Build history of the part. All positions in model axes, mm. Round coordinates to 2 decimals unless told otherwise and drop trailing zeros. Loops run counter-clockwise (first coordinate to the right, second up) from the corner with the lowest first, then second, coordinate; pieces in that order, holes last. Notation, with made-up numbers: M 6,-12.5 L 44,-12.5 A23 cw 44,23.5 Z; hole C -14.75,-4 d7. An arc over 180 degrees is marked long. One line per item, written item: value.
```python
from build123d import *

# Parameters (mm, degrees)
SKETCH4_R           = 1.0999978
BOSS_EXTRUDE4_DEPTH = 3.175
SKETCH1_R           = 1.1999976
CUT_EXTRUDE7_DEPTH  = 62.35209393
CUT_EXTRUDE9_DEPTH  = 62.35209393
CIRPATTERN1_COUNT   = 3
SKETCH9_W           = 40.35933
SKETCH9_H           = 5.08
BOSS_EXTRUDE5_DEPTH = 3.175
SKETCH10_R          = 1.2
CUT_EXTRUDE10_DEPTH = 64.132493246
CIRPATTERN2_COUNT   = 3
FILLET3_R           = 20.32
FILLET4_R           = 2.54
SKETCH13_W          = 6.35
SKETCH13_H          = 6.35
CUT_EXTRUDE12_DEPTH = 63.881962359


with BuildPart() as part:
    # Sketch4 → Boss-Extrude4 (new body)
    with BuildSketch(Plane(origin=(0, 0, 0), x_dir=(1, 0, 0), z_dir=(0, 1, 0))):
        with BuildLine():
            Line((-19.99996, 34.84845233), (-40.179625, -0.10375273))
            ThreePointArc((-40.179625, -0.10375273), (-38.616778752, -22.295407608), (-20.179665, -34.744699599))
            Line((-20.179665, -34.744699599), (0, -34.744699599))
            Line((0, -34.744699599), (20.179665, -34.744699599))
            ThreePointArc((20.179665, -34.744699599), (38.616778752, -22.295407608), (40.179625, -0.10375273))
            Line((40.179625, -0.10375273), (30.0897925, 17.3723498))
            Line((30.0897925, 17.3723498), (19.99996, 34.84845233))
            ThreePointArc((19.99996, 34.84845233), (0, 44.590815215), (-19.99996, 34.84845233))
        make_face()
        with Locations(Location((-5.000000033, 0, 0), (0, 0, 270))):
            Circle(SKETCH4_R, mode=Mode.SUBTRACT)
        with Locations(Location((5.000000033, 0, 0), (0, 0, 270))):
            Circle(SKETCH4_R, mode=Mode.SUBTRACT)
    extrude(amount=BOSS_EXTRUDE4_DEPTH)

    # Sketch1 → Cut-Extrude7 (cut, through all)
    with BuildSketch(Plane(origin=(0, 3.175, 0), x_dir=(1, 0, 0), z_dir=(0, 1, 0))):
        with Locations(Location((10.835999918, -25.497765942, 0), (0, 0, 270))):
            Circle(SKETCH1_R)
        with Locations(Location((10.835999918, -7.497801942, 0), (0, 0, 270))):
            Circle(SKETCH1_R)
        with Locations(Location((-11.911286913, -5.635350233, 0), (0, 0, 270))):
            Circle(SKETCH1_R)
        with Locations(Location((-27.499713005, 3.364631767, 0), (0, 0, 270))):
            Circle(SKETCH1_R)
        with Locations(Location((1.075286995, 13.133152175, 0), (0, 0, 270))):
            Circle(SKETCH1_R)
        with Locations(Location((16.663713087, 22.133134175, 0), (0, 0, 270))):
            Circle(SKETCH1_R)
    extrude(amount=-CUT_EXTRUDE7_DEPTH, mode=Mode.SUBTRACT)

    # Sketch6 → Cut-Extrude9 (cut, through all)
    with BuildSketch(Plane(origin=(0, 3.175, 0), x_dir=(1, 0, 0), z_dir=(0, 1, 0))):
        with BuildLine():
            Line((-20.179665, -31.862440942), (20.179665, -31.862440942))
            ThreePointArc((20.179665, -31.862440942), (20.554442, -31.487663942), (20.179665, -31.112886942))
            Line((20.179665, -31.112886942), (-20.179665, -31.112886942))
            ThreePointArc((-20.179665, -31.112886942), (-20.554442, -31.487663942), (-20.179665, -31.862440942))
        make_face()
    cut_extrude9 = extrude(amount=-CUT_EXTRUDE9_DEPTH, mode=Mode.SUBTRACT)

    # CirPattern1: Cut-Extrude9 ×3 about axis
    cirpattern1_axis = Axis((0, 0, -0.195474675), (0, 1, 0))
    for i in range(1, CIRPATTERN1_COUNT):
        add(cut_extrude9.rotate(cirpattern1_axis, i * 360 / CIRPATTERN1_COUNT), mode=Mode.SUBTRACT)

    # Sketch9 → Boss-Extrude5 (add)
    with BuildSketch(Plane(origin=(0, 3.175, 0), x_dir=(1, 0, 0), z_dir=(0, 1, 0))):
        Polygon((-19.99996, 34.84845233), (-24.399369051, 37.38845233), (-44.579034051, 2.43624727), (-40.179625, -0.10375273), align=None)
        with Locations((0, -37.284699599)):
            Rectangle(SKETCH9_W, SKETCH9_H)
        Polygon((19.99996, 34.84845233), (24.399369051, 37.38845233), (44.579034051, 2.43624727), (40.179625, -0.10375273), align=None)
    extrude(amount=-BOSS_EXTRUDE5_DEPTH)

    # Sketch10 → Cut-Extrude10 (cut, through all)
    with BuildSketch(Plane(origin=(0, 3.175, 0), x_dir=(1, 0, 0), z_dir=(0, 1, 0))):
        with Locations(Location((-32.140098419, 18.556094474, 0), (0, 0, 270))):
            Circle(SKETCH10_R)
    cut_extrude10 = extrude(amount=-CUT_EXTRUDE10_DEPTH, mode=Mode.SUBTRACT)

    # CirPattern2: Cut-Extrude10 ×3 about axis
    cirpattern2_axis = Axis((0.026468548, 0, 0.018558184), (0, 1, 0))
    for i in range(1, CIRPATTERN2_COUNT):
        add(cut_extrude10.rotate(cirpattern2_axis, i * 360 / CIRPATTERN2_COUNT), mode=Mode.SUBTRACT)

    # Fillet3
    # the kernel refuses this fillet: 20.32 mm, written as the material it adds along each edge
    with BuildSketch(Plane(origin=(-19.99996, 0, -34.84845233), x_dir=(0.7399559261961443, 0, -0.6726553555032522), z_dir=(0, 1, 0)), Plane(origin=(-20.179665, 0, 34.744699599), x_dir=(-0.9525145889555402, 0, -0.3044929520150809), z_dir=(0, 1, 0))) as fillet3_piece_1:
        with BuildLine():
            CenterArc((11.947307306, 20.031233261), FILLET3_R, 228.388118158, 31.941023553)
            Line((-1.546824196, 4.838774112), (-1.816706826, 4.534924929))
            ThreePointArc((-1.816706826, 4.534924929), (-1.160514027, 2.29564112), (-0.387101929, -0.123745936))
            Line((-0.387101929, -0.123745936), (0.068270327, -0.400624665))
            ThreePointArc((0.068270327, -0.400624665), (4.266895466, -0.045441577), (8.465520605, -0.400624665))
            Line((8.465520605, -0.400624665), (8.533790933, 0))
        make_face()
    extrude(amount=3.175)
    with BuildSketch(Plane(origin=(19.99996, 0, -34.84845233), x_dir=(-0.7399559261961431, 0, -0.6726553555032532), z_dir=(0, 1, 0)), Plane(origin=(20.179665, 0, 34.744699599), x_dir=(0.9525145889555428, 0, -0.3044929520150728), z_dir=(0, 1, 0))) as fillet3_piece_2:
        with BuildLine():
            CenterArc((11.947307306, -20.031233261), FILLET3_R, 99.67085829, 31.941023553)
            Line((-1.546824196, -4.838774112), (-1.816706826, -4.534924929))
            ThreePointArc((-1.816706826, -4.534924929), (-1.160514027, -2.29564112), (-0.387101929, 0.123745936))
            Line((-0.387101929, 0.123745936), (0.068270327, 0.400624665))
            ThreePointArc((0.068270327, 0.400624665), (4.266895466, 0.045441577), (8.465520605, 0.400624665))
            Line((8.465520605, 0.400624665), (8.533790933, 0))
        make_face()
    extrude(amount=3.175)
    with BuildSketch(Plane(origin=(40.179625, 0, 0.10375273), x_dir=(0.8660254037844389, 0, -0.4999999999999995), z_dir=(0, 1, 0))) as fillet3_piece_3:
        with BuildLine():
            CenterArc((15.442171046, -17.479353856), FILLET3_R, 120.660456863, 31.941023553)
            Line((-2.598479193, -8.128560362), (-2.959292198, -7.941544493))
            ThreePointArc((-2.959292198, -7.941544493), (-1.342523361, -4.050443541), (-0.402388672, 0.056958904))
            Line((-0.402388672, 0.056958904), (0, 0.4064))
            ThreePointArc((0, 0.4064), (2.54, 0.4064), (4.872756579, 0.349587077))
            Line((4.872756579, 0.349587077), (5.08, 0))
        make_face()
    extrude(amount=3.175)
    with BuildSketch(Plane(origin=(-40.179625, 0, 0.10375273), x_dir=(-0.8660254037844382, 0, -0.500000000000001), z_dir=(0, 1, 0))) as fillet3_piece_4:
        with BuildLine():
            CenterArc((15.442171046, 17.479353856), FILLET3_R, 207.398519584, 31.941023553)
            Line((-2.598479193, 8.128560362), (-2.959292198, 7.941544493))
            ThreePointArc((-2.959292198, 7.941544493), (-1.342523361, 4.050443541), (-0.402388672, -0.056958904))
            Line((-0.402388672, -0.056958904), (0, -0.4064))
            ThreePointArc((0, -0.4064), (2.54, -0.4064), (4.872756579, -0.349587077))
            Line((4.872756579, -0.349587077), (5.08, 0))
        make_face()
    extrude(amount=3.175)

    # Fillet4
    fillet4_edges = [part.edges().sort_by_distance(p)[0] for p in [
        (-44.579034051, 1.5875, -2.43624727),
        (-24.399369051, 1.5875, -37.38845233),
        (20.179665, 1.5875, 39.824699599),
        (-20.179665, 1.5875, 39.824699599),
        (24.399369051, 1.5875, -37.38845233),
        (44.579034051, 1.5875, -2.43624727),
    ]]
    fillet(fillet4_edges, radius=FILLET4_R)

    # Sketch13 → Cut-Extrude12 (cut, through all)
    with BuildSketch(Plane(origin=(0, 3.175, 0), x_dir=(1, 0, 0), z_dir=(0, 1, 0))):
        Rectangle(SKETCH13_W, SKETCH13_H)
    extrude(amount=-CUT_EXTRUDE12_DEPTH, mode=Mode.SUBTRACT)


solid = part.part
```
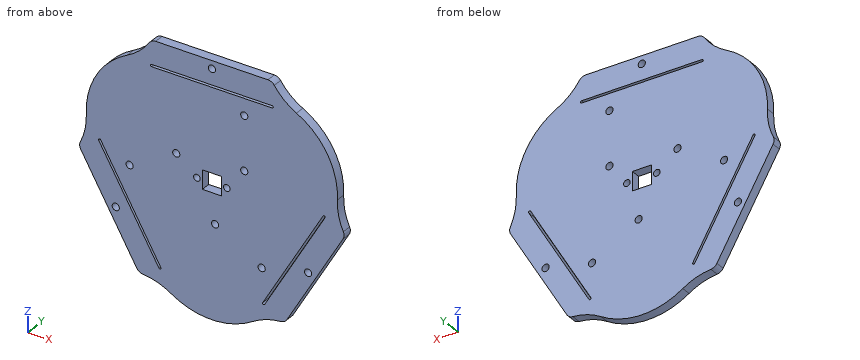
Item 1: Wall check: line 1 along X through (y, z) = (1.2, -10); line 2 along Z through (x, y) = (-12, 2.7); line 3 along Z through (x, y) = (-4, 1.35). Give the ranges that are in metal, low to high.
Check values:
line 1: x = -40.21 to -31.36, -30.49 to 30.49, 31.36 to 40.21
line 2: z = -41.58 to 4.44, 6.83 to 31.11, 31.86 to 39.82
line 3: z = -44.27 to -0.46, 0.46 to 31.11, 31.86 to 39.82
Item 2: Slice it at C-C, the plane z = 0. Give the cut face in (x, y) (3 decimals), and give its area (3 significant figures).
Check values:
outline: M -43.415,0 L -37.13,0 L -37.13,3.175 L -43.415,3.175 Z; M -36.265,0 L -6.1,0 L -6.1,3.175 L -36.265,3.175 Z; M -3.9,0 L -3.175,0 L -3.175,3.175 L -3.9,3.175 Z; M 3.175,0 L 3.9,0 L 3.9,3.175 L 3.175,3.175 Z; M 6.1,0 L 36.265,0 L 36.265,3.175 L 6.1,3.175 Z; M 37.13,0 L 43.415,0 L 43.415,3.175 L 37.13,3.175 Z
area: 236 mm2
Item 3: Drop flat-ended pins along their axis: P1, Ø1.9, axis at x = 10.84, z = 25.5, coming from the -Y side; P2, Ø1, axis at y = 2, z = 27, coming from the -X side; P3, Ø1.5, axis at x = 23, y = 1, coming from the +Z side; P4, Ø1.5, axis at y = 0.5, z = 25, coming from the +X side. Give the stop position or say it passes through.
Check values:
P1: passes through
P2: stops at x = -35.58
P3: stops at z = 36.94
P4: stops at x = 37.37
Item 4: Slice it at D-D, the plane y = 0.7. Give the number of separate pieces and of enclosed holes in the cut face, and give its area (3 significant figures).
Check values:
separate pieces: 1
enclosed holes: 15
area: 5,520 mm2
Item 5: Slice it at B-B, the plane x = -5. Give the cut face in (y, z) (3 decimals).
Check values:
outline: M 0,-44.094 L 3.175,-44.094 L 3.175,-1.1 L 0,-1.1 Z; M 0,1.1 L 3.175,1.1 L 3.175,31.113 L 0,31.113 Z; M 0,31.862 L 3.175,31.862 L 3.175,39.825 L 0,39.825 Z
Item 6: Slice it at A-A, the plane z = -25.5. Give the cut face in (x, y) (3 decimals).
Check values:
outline: M -31.263,0 L -22.408,0 L -22.408,3.175 L -31.263,3.175 Z; M -21.542,0 L 21.542,0 L 21.542,3.175 L -21.542,3.175 Z; M 22.408,0 L 31.263,0 L 31.263,3.175 L 22.408,3.175 Z
